Verification items for this drawing (mm, ordinates from the low corner). A direction names the side the tool comes from. Round coordinates to 2 decimals unless told otherwise and drop trailing zeros. Loops run counter-clockwise (first coordinate to the right, second up) from the corner with the lowest first, then second, coordinate; pieces in that order, holes last. Notation, with made-up numbers: M 36.25,-28 L 68.25,-28 A11 cw 68.25,-22 Z; hole C 58,88.5 d4. An arc over 180 degrees is marked long. Use one line per item in the form item = value. Start each with the question number.
1. Material ranges on line 1 (Z direction, x = 4.75, y = 2), recorded low to high.
2. Draft check along Y on the marked faces 1, 2 and 3. Enter one of: pulls with the +Y half, pulls with the -Y half, needs draft (parallel to the pull), parting line crosses it, or undercut.
3. Cross-section at D-D (x = 12.25). Record the boundary of the cut face in (y, z).
4. Cross-section at C-C (z = 10.5). Record the boundary of the cut face in (x, y).
5. Set-up check for the marked faces 4 and 5: record each of +Z, -Z, +X, -X, +Y, -Y from which the full face is reachable in a straight line by a thin tool's end or side.
6. Go/stop test with flat-tipped pins: pin 1 (1 mm diameter, centred on x = 6, y = 15, fed in from +Z); pin 2 (6 mm diameter, centred on x = 5, z = 13, fed in from +Y). Record where each tip stops, or that it passes through.
7. Cross-section at A-A (y = 10). Record the boundary of the cut face in (x, z).
8. Cross-section at B-B (x = 10). Record the boundary of the cut face in (y, z).
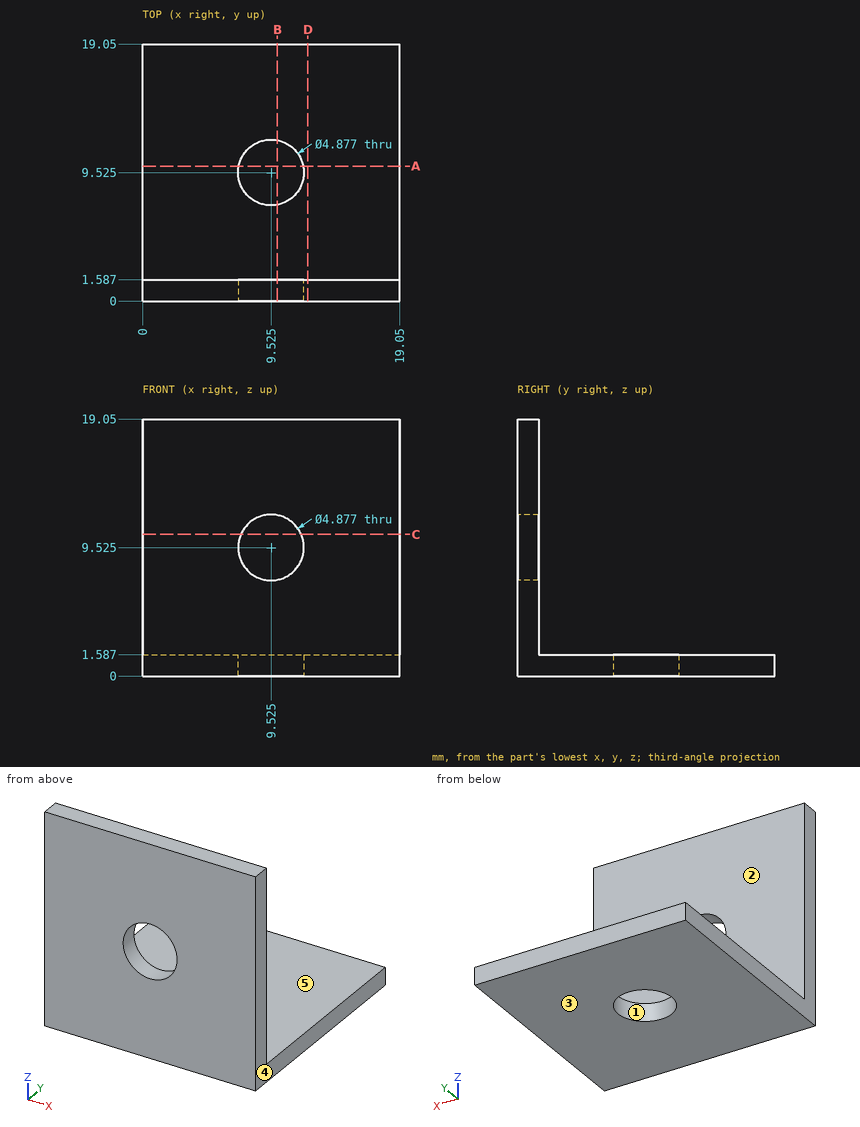
Reported:
q1.line_1 = 0 to 1.59
q2.face_1 = undercut
q2.face_2 = pulls with the +Y half
q2.face_3 = needs draft
q3.outline = M 0,0 L 19.05,0 L 19.05,1.59 L 1.59,1.59 L 1.59,19.05 L 0,19.05 Z
q4.outline = M 0,0 L 7.29,0 L 7.29,1.59 L 0,1.59 Z; M 11.76,0 L 19.05,0 L 19.05,1.59 L 11.76,1.59 Z
q5.face_4 = +Z, -Z, +X, +Y, -Y
q5.face_5 = +Z, +X, -X, +Y
q6.pin_1 = 1.59
q6.pin_2 = 1.59
q7.outline = M 0,0 L 7.13,0 L 7.13,1.59 L 0,1.59 Z; M 11.92,0 L 19.05,0 L 19.05,1.59 L 11.92,1.59 Z
q8.outline = M 0,0 L 7.13,0 L 7.13,1.59 L 1.59,1.59 L 1.59,7.13 L 0,7.13 Z; M 0,11.92 L 1.59,11.92 L 1.59,19.05 L 0,19.05 Z; M 11.92,0 L 19.05,0 L 19.05,1.59 L 11.92,1.59 Z
